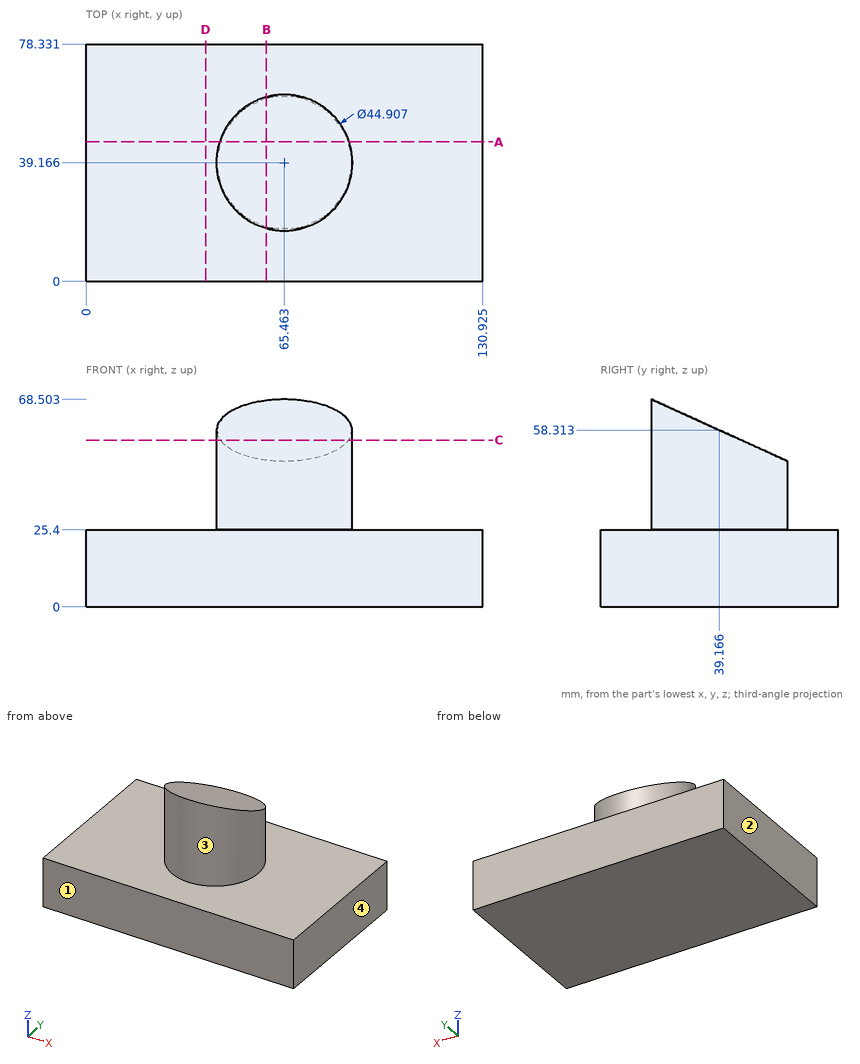
The drawing under review shows one solid part. Ordinate dimensions are in mm from its lowest x, y, z. Give positions to 0.01 mm unless a question says otherwise; leave off trailing zeros. Write each loop counter-clockwise with the first axis right and the second up, starting at its lowest first coordinate (ties: lowest second). Pieces come first, ordered by that corner, then holes. Notation, with made-up numbers: (-35.75, 32) -> (3.25, 32) arc R9 ccw to (3.25, 43) -> close; hole circle Ø6 at (27, 41.5). An arc over 180 degrees is marked (long way). Use CSV: the item, a comma, the result in double quotes.
Q1. To check wall thickness, follow probe 1 along Z at (x, y) = (40.5, 21); probe 2 along Y at (x, z) = (65, 34.5) (1 decimal); probe 3 along Z at (x, y) = (61, 25). State the ranges of each line that lie inside material, in increasing order. Write a range as [from, to].
Conclusion:
probe 1,"[0, 25.4]"
probe 2,"[16.7, 61.6]"
probe 3,"[0, 64.74]"
Q2. Take a section at A-A, the plane y = 46. Write out the cut boundary in (x, z) (1 decimal), then the cut area to 3 significant figures.
Conclusion:
outline,"(0, 0) -> (130.9, 0) -> (130.9, 25.4) -> (86.9, 25.4) -> (86.9, 55.2) -> (44.1, 55.2) -> (44.1, 25.4) -> (0, 25.4) -> close"
area,"4,600 mm2"
Q3. Mouldability with a two-part tool opening along X and no side actions: class the marked faces 1, 2, 3 and 4 as pulls with the +X half, pulls with the -X half, needs draft (parallel to the pull), parting line crosses it, or undercut.
Conclusion:
face 1,"needs draft"
face 2,"pulls with the -X half"
face 3,"parting line crosses it"
face 4,"pulls with the +X half"
Q4. For P1, Ø12, axis at x = 21, z = 30.5, coming from the +Y side; P2, Ø3, axis at y = 27, z = 33.5, coming from the +X side; P3, Ø10, axis at x = 18.5, y = 49, coming from the +Z side; P4, Ø4, axis at x = 81.5, z = 41.5, coming from the -Y side, all flat-tipped, find the tip position at first contact; note any pin that passes through.
Conclusion:
P1,"y = 78.33"
P2,"x = 85.22"
P3,"z = 25.4"
P4,"y = 21.64"
Q5. Take a section at C-C, the plane z = 55. Write out the cut boundary in (x, y) (1 decimal).
Conclusion:
outline,"(44.2, 46.5) arc R22.5 ccw (long way) to (86.7, 46.5) -> close"
Q6. Take a section at B-B, the plane x = 59.5. Write out the cut boundary in (y, z).
Conclusion:
outline,"(0, 0) -> (78.33, 0) -> (78.33, 25.4) -> (60.81, 25.4) -> (60.81, 48.49) -> (17.52, 68.14) -> (17.52, 25.4) -> (0, 25.4) -> close"
Q7. Take a section at D-D, the plane x = 39.5. Write out the cut boundary in (y, z).
Conclusion:
outline,"(0, 0) -> (78.33, 0) -> (78.33, 25.4) -> (0, 25.4) -> close"
